```python
from build123d import *

# Parameters (mm, degrees)
SKICA1_W                    = 67
SKICA1_H                    = 50
P_IDAT_VYSUNUT_M1_DEPTH     = 3
ODEBRAT_VYSUNUT_M1_DEPTH    = 1
SKICA3_W                    = 8
SKICA3_H                    = 8
ODEBRAT_VYSUNUT_M2_DEPTH    = 4
VYSUNOUT_TENKOST_NN_1_DEPTH = 1
VYSUNOUT_TENKOST_NN_2_DEPTH = 5
SKICA6_W                    = 12
SKICA6_H                    = 4
ODEBRAT_VYSUNUT_M3_DEPTH    = 4
ODEBRAT_VYSUNUT_M5_DEPTH    = 1
P_IDAT_START                = -1
P_IDAT_VYSUNUT_M5_DEPTH     = 1
P_IDAT_VYSUNUT_M6_DEPTH     = 1
ODEBRAT_VYSUNUT_M6_DEPTH    = 1
SKICA13_W                   = 1.825387876
SKICA13_H                   = 1.792199005
P_IDAT_VYSUNUT_M7_DEPTH     = 1


with BuildPart() as part:
    # Skica1 → Přidat vysunutím1 (new body)
    with BuildSketch(Plane.XY):
        Rectangle(SKICA1_W, SKICA1_H)
    extrude(amount=P_IDAT_VYSUNUT_M1_DEPTH)

    # Skica2 → Odebrat vysunutím1 (cut)
    with BuildSketch(Plane.XY.offset(3)):
        Polygon((-25.5, -22), (-30.5, -17), (-30.5, 17), (-25.5, 22), (25.5, 22), (30.5, 17), (30.5, -17), (25.5, -22), align=None)
    extrude(amount=-ODEBRAT_VYSUNUT_M1_DEPTH, mode=Mode.SUBTRACT)

    # Skica3 → Odebrat vysunutím2 (cut, through all)
    with BuildSketch(Plane(origin=(0, 0, 0), x_dir=(-1, 0, 0), z_dir=(0, 0, -1))):
        with Locations((20, -3)):
            Rectangle(SKICA3_W, SKICA3_H)
        with Locations((-20, -3)):
            Rectangle(SKICA3_W, SKICA3_H)
        Polygon((25.5, -25), (-25.5, -25), (-25.5, -12), (-12, -12), (-12, 15), (12, 15), (12, -12), (25.5, -12), align=None)
    extrude(amount=-ODEBRAT_VYSUNUT_M2_DEPTH, mode=Mode.SUBTRACT)

    # Skica4 → Vysunout tenkostěnný1 (add)
    with BuildSketch(Plane.XY.offset(2)):
        Polygon((-12, -12), (-12, 15), (12, 15), (12, -12), (13, -12), (13, 16), (-13, 16), (-13, -12), align=None)
    extrude(amount=VYSUNOUT_TENKOST_NN_1_DEPTH)

    # Skica5 → Vysunout tenkostěnný2 (add)
    with BuildSketch(Plane(origin=(0, 0, 0), x_dir=(-1, 0, 0), z_dir=(0, 0, -1))):
        Polygon((-25.5, -25), (-33.5, -25), (-33.5, 25), (33.5, 25), (33.5, -25), (25.5, -25), (25.5, -26), (34.5, -26), (34.5, 26), (-34.5, 26), (-34.5, -26), (-25.5, -26), align=None)
    extrude(amount=-VYSUNOUT_TENKOST_NN_2_DEPTH)

    # Skica6 → Odebrat vysunutím3 (cut, through all)
    with BuildSketch(Plane.XY.offset(2)):
        with Locations((0, 24)):
            Rectangle(SKICA6_W, SKICA6_H)
    extrude(amount=ODEBRAT_VYSUNUT_M3_DEPTH, mode=Mode.SUBTRACT)

    # Skica7 → Odebrat vysunutím5 (cut)
    with BuildSketch(Plane(origin=(0, 0, 0), x_dir=(-1, 0, 0), z_dir=(0, 0, -1))):
        Polygon((-32.44, 14.540476732), (-23.459523268, 23.94), (-14.06, 14.959523268), (-23.040476732, 5.56), align=None)
        Polygon((14.06, 14.959523268), (23.040476732, 5.56), (32.44, 14.540476732), (23.459523268, 23.94), align=None)
    extrude(amount=-ODEBRAT_VYSUNUT_M5_DEPTH, mode=Mode.SUBTRACT)

    # Skica8 → Přidat vysunutím5 (add)
    with BuildSketch(Plane(origin=(0, 0, 0), x_dir=(-1, 0, 0), z_dir=(0, 0, -1)).offset(P_IDAT_START)):
        with BuildLine():
            Line((-29.266904741, 14.966465555), (-25.766904741, 15.0801236))
            add(Edge.make_bspline(
                [(-29.266904741, 14.966465555), (-27.398369795, 11.364860762), (-25.766904741, 15.0801236)],
                knots=[0, 0, 0, 1, 1, 1], degree=2))
        make_face()
        with BuildLine():
            Line((-23.70327201, 17.257603785), (-23.747591798, 20.757603785))
            add(Edge.make_bspline(
                [(-23.70327201, 17.257603785), (-20.063848901, 19.047335046), (-23.747591798, 20.757603785)],
                knots=[0, 0, 0, 1, 1, 1], degree=2))
        make_face()
        with BuildLine():
            Line((29.266904741, 14.966465555), (25.766904741, 15.0801236))
            add(Edge.make_bspline(
                [(29.266904741, 14.966465555), (27.398369795, 11.364860762), (25.766904741, 15.0801236)],
                knots=[0, 0, 0, 1, 1, 1], degree=2))
        make_face()
        with BuildLine():
            Line((23.70327201, 17.257603785), (23.747591798, 20.757603785))
            add(Edge.make_bspline(
                [(23.70327201, 17.257603785), (20.063848901, 19.047335046), (23.747591798, 20.757603785)],
                knots=[0, 0, 0, 1, 1, 1], degree=2))
        make_face()
    extrude(amount=P_IDAT_VYSUNUT_M5_DEPTH)

    # Skica11 → Přidat vysunutím6 (add)
    with BuildSketch(Plane(origin=(0, 0, 0), x_dir=(-1, 0, 0), z_dir=(0, 0, -1)).offset(P_IDAT_START)):
        Polygon((-25.724541131, 9.230843392), (-24.69196981, 9.842232358), (-24.987531509, 11.719102967), (-22.99084361, 11.83415701), (-22.744580902, 14.120935241), (-20.448389818, 14.25324739), (-20.234248333, 16.2417502), (-18.334248333, 16.35123285), (-17.798682715, 17.425090135), (-17.654074665, 17.286928954), (-17.037308405, 14.35101353), (-18.237308405, 14.35101353), (-18.595837474, 12.383411714), (-20.461373652, 12.023169065), (-20.664808063, 10.134091396), (-22.628530356, 9.754888608), (-22.628530356, 8.554888608), (-25.57993308, 9.092682212), align=None)
        Polygon((22.628530356, 8.554888608), (25.57993308, 9.092682212), (25.724541131, 9.230843392), (24.69196981, 9.842232358), (24.987531509, 11.719102967), (22.99084361, 11.83415701), (22.744580902, 14.120935241), (20.448389818, 14.25324739), (20.234248333, 16.2417502), (18.334248333, 16.35123285), (17.798682715, 17.425090135), (17.654074665, 17.286928954), (17.037308405, 14.35101353), (18.237308405, 14.35101353), (18.595837474, 12.383411714), (20.461373652, 12.023169065), (20.664808063, 10.134091396), (22.628530356, 9.754888608), align=None)
    extrude(amount=P_IDAT_VYSUNUT_M6_DEPTH)

    # Skica12 → Odebrat vysunutím6 (cut)
    with BuildSketch(Plane(origin=(0, 0, 0), x_dir=(-1, 0, 0), z_dir=(0, 0, -1))):
        Polygon((-10.16, 23.3), (-6.369480049, 23.3), (-6.369480049, 22.56693444), (-5.70000808, 22.56693444), (-5.70000808, 20.774735435), (-6.347191054, 20.774735435), (-6.347191054, 20.077769155), (-6.944590723, 20.077769155), (-6.944590723, 19.546747227), (-6.347191054, 19.546747227), (-6.347191054, 18.733619901), (-5.70000808, 18.733619901), (-5.70000808, 17.804331528), (-7.143723945, 17.804331528), (-7.143723945, 18.501297807), (-7.774312484, 18.501297807), (-7.774312484, 19.140183564), (-8.253595527, 19.140183564), (-8.253595527, 20.077769155), (-8.769978599, 20.077769155), (-8.769978599, 17.804331528), (-10.16, 17.804331528), align=None)
        Polygon((-4.936617449, 23.3), (-3.432005952, 23.3), (-3.432005952, 18.733619901), (-1.815348918, 18.733619901), (-1.815348918, 23.3), (-0.352474449, 23.3), (-0.352474449, 18.501297807), (-1.072767186, 18.501297807), (-1.072767186, 17.804331528), (-4.258061738, 17.804331528), (-4.258061738, 18.501297807), (-4.936617449, 18.501297807), align=None)
        Polygon((4.306009733, 22.56693444), (4.967857854, 22.56693444), (4.967857854, 21.583119882), (3.37998692, 21.583119882), (3.37998692, 22.255759653), (1.9023848, 22.255759653), (1.9023848, 21.01680995), (4.251110557, 21.01680995), (4.251110557, 20.304001629), (4.967857854, 20.304001629), (4.967857854, 18.501297807), (4.251110557, 18.501297807), (4.251110557, 17.804331528), (1.031261162, 17.804331528), (1.031261162, 18.501297807), (0.42478268, 18.501297807), (0.42478268, 19.546747227), (1.9023848, 19.546747227), (1.9023848, 18.820740686), (3.468201971, 18.820740686), (3.468201971, 20.077769155), (1.031261162, 20.077769155), (1.031261162, 20.774735435), (0.42478268, 20.774735435), (0.42478268, 22.56693444), (1.031261162, 22.56693444), (1.031261162, 23.3), (4.306009733, 23.3), align=None)
        Polygon((5.672754202, 23.3), (7.173807496, 23.3), (7.173807496, 21.079366958), (8.764209199, 21.079366958), (8.764209199, 23.3), (10.1580444, 23.3), (10.1580444, 17.804331528), (8.764209199, 17.804331528), (8.764209199, 20.077769155), (7.173807496, 20.077769155), (7.173807496, 17.804331528), (5.672754202, 17.804331528), align=None)
    extrude(amount=-ODEBRAT_VYSUNUT_M6_DEPTH, mode=Mode.SUBTRACT)

    # Skica13 → Přidat vysunutím7 (add)
    with BuildSketch(Plane(origin=(0, 0, 0), x_dir=(-1, 0, 0), z_dir=(0, 0, -1)).offset(P_IDAT_START)):
        with Locations((-7.857284661, 21.670834938)):
            Rectangle(SKICA13_W, SKICA13_H)
    extrude(amount=P_IDAT_VYSUNUT_M7_DEPTH)


solid = part.part
```
CAD build for the part. Positions are in the model's coordinates, mm. A direction names the side the tool comes from. Give positions to 0.01 mm unless a question says otherwise; leave off trailing zeros. Loops run counter-clockwise (first coordinate to the right, second up) from the corner with the lowest first, then second, coordinate; pieces in that order, holes last. Notation, with made-up numbers: (-39, 0.25) -> (5, 0.25) arc R16 ccw to (5, 30.25) -> close; hole circle Ø9 at (-37, -2.5). An arc over 180 degrees is marked (long way). Use a Markdown table: item, result.
1. Slice it at B-B (z = 4.2). List the corners of the cut face in (x, y).
Check result:
| item | result |
|---|---|
| outline | (-34.5, -26) -> (-25.5, -26) -> (-25.5, -25) -> (-33.5, -25) -> (-33.5, 25) -> (-6, 25) -> (-6, 26) -> (-34.5, 26) -> close; (6, 25) -> (33.5, 25) -> (33.5, -25) -> (25.5, -25) -> (25.5, -26) -> (34.5, -26) -> (34.5, 26) -> (6, 26) -> close |
2. Mould opens along X. For faces 1 (the flat face through (-23, 15, 1)), 2 (the flat face through (0, 15, 1)), 3 (the flat face through (-34, 12, 5)) say: pulls with the +X half, pulls with the -X half, needs draft (parallel to the pull), parting line crosses it, or undercut.
Check result:
| item | result |
|---|---|
| face 1 | undercut |
| face 2 | undercut |
| face 3 | needs draft |
3. Slice it at A-A (y = -8). List the corners of the cut face in (x, z), plus the area to 3 significant figures.
Check result:
| item | result |
|---|---|
| outline | (-34.5, 0) -> (-12, 0) -> (-12, 3) -> (-13, 3) -> (-13, 2) -> (-30.5, 2) -> (-30.5, 3) -> (-33.5, 3) -> (-33.5, 5) -> (-34.5, 5) -> close; (12, 0) -> (34.5, 0) -> (34.5, 5) -> (33.5, 5) -> (33.5, 3) -> (30.5, 3) -> (30.5, 2) -> (13, 2) -> (13, 3) -> (12, 3) -> close |
| area | 104 mm^2 |
4. Flat gauge pins, fed straight in: pin 1 (2 mm diameter, centred on x = 27, y = 6.5, fed in from -Z); pin 2 (2 mm diameter, centred on x = -3.5, z = 3.5, fed in from +Y); pin 3 (8 mm diameter, centred on x = -26, y = 0, fed in from +Z); pin 4 (0.6 mm diameter, centred on x = -4.5, z = 0.5, fed in from -Y). Where does each tip first touch, or does it go through?
Check result:
| item | result |
|---|---|
| pin 1 | stops at z = 0 |
| pin 2 | stops at y = 16 |
| pin 3 | stops at z = 2 |
| pin 4 | stops at y = 15 |
5. Wall check: L1, parallel to X at y = -6, z = 1.9; L2, parallel to X at y = -5, z = 2.2; L3, parallel to X at y = 24.5, z = 4. Give the ranges that are in metal, low to high. Write a range as [from, to].
Check result:
| item | result |
|---|---|
| L1 | x = [-34.5, -24], [-16, -12], [12, 16], [24, 34.5] |
| L2 | x = [-34.5, -30.5], [-13, -12], [12, 13], [30.5, 34.5] |
| L3 | x = [-34.5, -33.5], [33.5, 34.5] |
6. Slice it at C-C (y = -19). List the corners of the cut face in (x, z).
Check result:
| item | result |
|---|---|
| outline | (-34.5, 0) -> (-25.5, 0) -> (-25.5, 2) -> (-28.5, 2) -> (-28.5, 3) -> (-33.5, 3) -> (-33.5, 5) -> (-34.5, 5) -> close; (25.5, 0) -> (34.5, 0) -> (34.5, 5) -> (33.5, 5) -> (33.5, 3) -> (28.5, 3) -> (28.5, 2) -> (25.5, 2) -> close |
7. Which spindle directions (+Z, -Z, +X, -X, +Y, -Y) get a long thin tool onto all of the face, cutting with end or side? Do faces 4 (the flat face through (-28, -19.5, 2.5)), 5 (the flat face through (-18.826, 19.513, 0.493)), 6 (the flat face through (-20, -7, 1)). Say none if no direction does.
Check result:
| item | result |
|---|---|
| face 4 | +Z |
| face 5 | -Z |
| face 6 | +Z, -Z |
